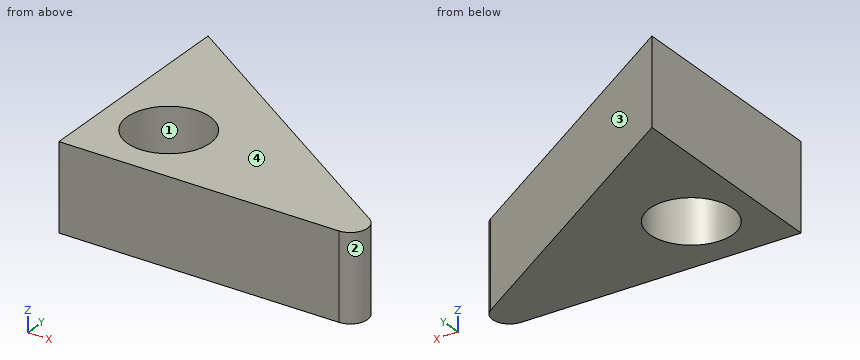
from build123d import *

# Parameters (mm, degrees)
F1_DEPTH = 25.4
F2_R     = 5.08
F3_R     = 12.218355
F4_DEPTH = 25.4


with BuildPart() as f1:
    # F0 (on Top) → F1 (new body)
    with BuildSketch(Plane.XY):
        Polygon((51.096436, -34.222286), (-48.252478, 31.188732), (-48.252478, -34.222286), align=None)
    extrude(amount=F1_DEPTH)

    # F2
    f2_edges = [f1.edges().sort_by_distance(p)[0] for p in [
        (51.096436, -34.222286, 12.7),
    ]]
    fillet(f2_edges, radius=F2_R)

    # F3 (on face) → F4 (cut)
    with BuildSketch(Plane.XY.offset(25.4)):
        with Locations((-29.29276, -14.314586)):
            Circle(F3_R)
    extrude(amount=-F4_DEPTH, mode=Mode.SUBTRACT)


solid = f1.part
Could you check a few things on this model? Use its own coordinates, in mm. Face numbers are marked on the shaded views. Round coordinates to 2 decimals unless told otherwise and drop trailing zeros. Order: outer loops, then holes, each group sorted by start corner. A loop starts at its lowest first (then second) coordinate and runs counter-clockwise, first axis right, second up.
(1) Imagine slicing it at B-B (x = -31). Write out the boundary of the cut face in (y, z), plus the area to 3 significant figures.
Response values:
outline: (-34.22, 0) - (-26.41, 0) - (-26.41, 25.4) - (-34.22, 25.4) - close; (-2.22, 0) - (19.83, 0) - (19.83, 25.4) - (-2.22, 25.4) - close
area: 758 mm2
(2) Imagine slicing it at D-D (x = -9.5). Write out the boundary of the cut face in (y, z), plus the area to 3 significant figures.
Response values:
outline: (-34.22, 0) - (5.67, 0) - (5.67, 25.4) - (-34.22, 25.4) - close
area: 1,010 mm2
(3) If we mould it in two halves opening along Y, with no side actions, what happens to the marked faces 1, 2, 3 and 4? For each: released by +Y, released by -Y, zero draft, split by the parting line, or undercut.
Response values:
face 1: undercut
face 2: split by the parting line
face 3: released by +Y
face 4: zero draft
(4) Please list where these lines run through material, in increasing order: line 1 along X through (y, z) = (-24, 16.75); line 2 along X through (y, z) = (-22, 10.75); line 3 along Y through (x, z) = (-36.5, 8).
Response values:
line 1: x = -48.25 to -36.74, -21.84 to 35.57
line 2: x = -48.25 to -38.79, -19.79 to 32.53
line 3: y = -34.22 to -24.18, -4.45 to 23.45
(5) Imagine slicing it at A-A (y = -15.5). Write out the boundary of the cut face in (x, z), plus the area to 3 significant figures.
Response values:
outline: (-48.25, 0) - (-41.45, 0) - (-41.45, 25.4) - (-48.25, 25.4) - close; (-17.13, 0) - (22.66, 0) - (22.66, 25.4) - (-17.13, 25.4) - close
area: 1,180 mm2
(6) I'm going to push flat-ended pins straight in: pin 1 (1 mm diameter, centred on x = -21.5, z = 7.5, fed in from +Y); pin 2 (1.5 mm diameter, centred on y = -12.5, z = 22, fed in from +X); pin 3 (4 mm diameter, centred on y = 4.5, z = 20.5, fed in from +X); pin 4 (14.5 mm diameter, centred on x = -29.29, y = -14.31, fed in from -Z). Where does each tip first touch, or does it pass through?
Response values:
pin 1: stops at y = 13.9
pin 2: stops at x = 19.24
pin 3: stops at x = -4.68
pin 4: passes through
(7) Imagine slicing it at C-C (z = 23.75). Write out the boundary of the cut face in (x, y).
Response values:
outline: (-48.25, -34.22) - (34.14, -34.22) arc R5.08 ccw to (36.94, -24.9) - (-48.25, 31.19) - close; hole circle Ø24.44 at (-29.29, -14.31)
